Design review of the part built by this model. Coordinates are the model's own, in mm. A direction names the side the tool comes from. Round coordinates to 2 decimals unless told otherwise and drop trailing zeros. Write each loop counter-clockwise with the first axis right and the second up, starting at its lowest first coordinate (ties: lowest second). Pieces come first, ordered by that corner, then holes. Notation, with made-up numbers: (-4.75, 78) - (16.25, 78) arc R13 ccw to (16.25, 87) - close; hole circle Ø8 at (82.5, -20.5). An arc over 180 degrees is marked (long way). Use one line per item in the form item = value.
```python
from build123d import *

# Parameters (mm, degrees)
SKETCH1_W           = 98.9
SKETCH1_H           = 90
SKETCH1_R           = 4
BOSS_EXTRUDE1_DEPTH = 5
SKETCH2_W           = 5
SKETCH2_H           = 90
BOSS_EXTRUDE2_DEPTH = 10
CHAMFER1_SIZE       = 2


with BuildPart() as part:
    # Sketch1 → Boss-Extrude1 (new body)
    with BuildSketch(Plane(origin=(0, 0, 0), x_dir=(1, 0, 0), z_dir=(0, 1, 0))):
        Rectangle(SKETCH1_W, SKETCH1_H)
        with Locations(Location((-37.875, -37.875, 0), (0, 0, 270))):
            Circle(SKETCH1_R, mode=Mode.SUBTRACT)
        with Locations(Location((37.875, -37.875, 0), (0, 0, 270))):
            Circle(SKETCH1_R, mode=Mode.SUBTRACT)
        with Locations(Location((-37.875, 37.875, 0), (0, 0, 270))):
            Circle(SKETCH1_R, mode=Mode.SUBTRACT)
        with BuildLine():
            Line((-25, 0), (0, 0))
            Line((0, 0), (0, 25))
            ThreePointArc((0, 25), (17.67766953, -17.67766953), (-25, 0))
        make_face(mode=Mode.SUBTRACT)
        with Locations(Location((37.875, 37.875, 0), (0, 0, 270))):
            Circle(SKETCH1_R, mode=Mode.SUBTRACT)
    extrude(amount=BOSS_EXTRUDE1_DEPTH)

    # Sketch2 → Boss-Extrude2 (add)
    with BuildSketch(Plane.XZ):
        with Locations((-46.95, 0)):
            Rectangle(SKETCH2_W, SKETCH2_H)
        with Locations((46.95, 0)):
            Rectangle(SKETCH2_W, SKETCH2_H)
    extrude(amount=BOSS_EXTRUDE2_DEPTH)

    # Chamfer1
    chamfer1_edges = [part.edges().sort_by_distance(p)[0] for p in [
        (-44.45, -10, 0),
        (44.45, -10, 0),
    ]]
    chamfer(chamfer1_edges, length=CHAMFER1_SIZE)


solid = part.part
```
Q1. For P1, Ø8, axis at x = -27.5, z = -18, coming from the -Y side, flat-tipped, find the tip position at first contact; note if it passes through.
Calculated:
P1 = 0
Q2. To check wall thickness, follow line 1 along X through (y, z) = (-1, 31.5); line 2 along Y through (x, z) = (-8.5, -39.5); line 3 along X through (y, z) = (-8.75, 25). State the ranges of each line that lie inside material, in increasing order. Write a range as from..to.
Calculated:
line_1 = -49.45..-44.45, 44.45..49.45
line_2 = 0..5
line_3 = -49.45..-45.2, 45.2..49.45
Q3. We need section B-B on x = 6. Write out the cut boundary in (y, z), then the cut area to 3 significant figures.
Calculated:
outline = (0, -45) - (5, -45) - (5, -24.27) - (0, -24.27) - close; (0, 24.27) - (5, 24.27) - (5, 45) - (0, 45) - close
area = 207 mm2
Q4. Draft analysis for pull direction Z (two halves, no side actions). For faces 4 (the flat face through (48, -10, 1)), 5 (the cylindrical face through (-33.91, 2.46, -38.4)), 6 (the flat face through (-12, 1, -45)), state which applies: released by +Z, released by -Z, zero draft, split by the parting line, or undercut.
Calculated:
face_4 = zero draft
face_5 = undercut
face_6 = released by -Z
Q5. Machinability: for faces 1 (the flat face through (-1, 5, -1)), 2 (the flat face through (44.45, -4, -1)), 3 (the flat face through (-13, 2, 0)), which of the approach directions +Z, -Z, +X, -X, +Y, -Y give a long, thin tool a straight path to every point of the face, cutting with its end or side? Answer none if there is none.
Calculated:
face_1 = +Z, -Z, +X, -X, +Y
face_2 = +Z, -Z, -Y
face_3 = +Y, -Y
Q6. We need section D-D on y = 2. Write out the cut boundary in (x, z) (3 decimals), then the cut area to 3 significant figures.
Calculated:
outline = (-49.45, -45) - (49.45, -45) - (49.45, 45) - (-49.45, 45) - close; hole circle Ø8 at (-37.875, -37.875); hole circle Ø8 at (-37.875, 37.875); hole (-25, 0) - (0, 0) - (0, -25) arc R25 ccw (long way) to start; hole circle Ø8 at (37.875, -37.875); hole circle Ø8 at (37.875, 37.875)
area = 7,230 mm2
Q7. We need section C-C on x = 35.5. Write out the cut boundary in (y, z).
Calculated:
outline = (0, -45) - (5, -45) - (5, -41.09) - (0, -41.09) - close; (0, -34.66) - (5, -34.66) - (5, 34.66) - (0, 34.66) - close; (0, 41.09) - (5, 41.09) - (5, 45) - (0, 45) - close
Q8. We need section A-A on y = -5.75. Write out the cut boundary in (x, z).
Calculated:
outline = (-49.45, -45) - (-44.45, -45) - (-44.45, 45) - (-49.45, 45) - close; (44.45, -45) - (49.45, -45) - (49.45, 45) - (44.45, 45) - close
